Source: three-view drawing plus pictorial views. Frame: mm from the lowest corner of the part. A direction names the side the tool comes from. Round coordinates to 2 decimals unless told otherwise and drop trailing zeros. Write each loop counter-clockwise with the first axis right and the second up, starting at its lowest first coordinate (ties: lowest second). Pieces come first, ordered by that corner, then holes. Notation, with made-up numbers: (5.25, 3) - (19.25, 3) arc R9 ccw to (19.25, 7) - close; hole circle Ø11 at (19, 54). An arc over 180 degrees is marked (long way). Write each question's results on one line, items separated by ' | '.
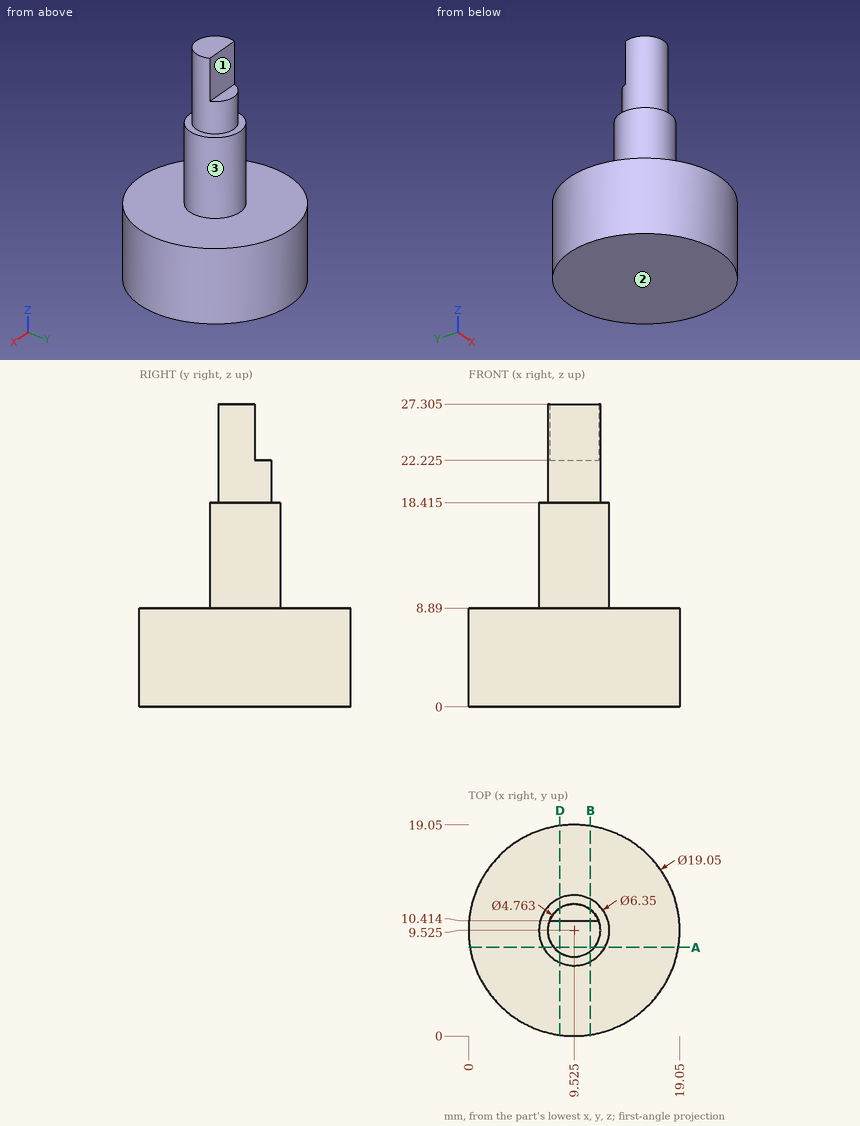
Q1. Section query D-D, the plane x = 8.25. Return loops of the section in (y, z) (1 decimal).
Answer block:
outline: (0.1, 0) - (19, 0) - (19, 8.9) - (12.4, 8.9) - (12.4, 18.4) - (11.5, 18.4) - (11.5, 22.2) - (10.4, 22.2) - (10.4, 27.3) - (7.5, 27.3) - (7.5, 18.4) - (6.6, 18.4) - (6.6, 8.9) - (0.1, 8.9) - close
Q2. Section query A-A, the plane y = 8. Return loops of the section in (x, z) (1 decimal).
Answer block:
outline: (0.1, 0) - (18.9, 0) - (18.9, 8.9) - (12.3, 8.9) - (12.3, 18.4) - (11.4, 18.4) - (11.4, 27.3) - (7.7, 27.3) - (7.7, 18.4) - (6.7, 18.4) - (6.7, 8.9) - (0.1, 8.9) - close
Q3. Access query for the marked faces 1, 2 and 3. Directions: +Z, -Z, +X, -X, +Y, -Y. A direction counts if a zero-diameter tool reaches every point of the face in a straight line with its end or side. Return the directions, or none.
Answer block:
face 1: +Z, +X, -X, +Y | face 2: -Z, +X, -X, +Y, -Y | face 3: +Z
Q4. Pin query (flat end, axial travel): pin 1 (6 mm diameter, centred on x = 4, z = 16.5, fed in from -Y); pin 2 (2 mm diameter, centred on x = 15, z = 19.5, fed in from -Y); pin 3 (3 mm diameter, centred on y = 5.5, z = 17.5, fed in from +X); pin 4 (1.2 mm diameter, centred on x = 10.5, y = 11.5, fed in from +Z) (1 decimal). Return the tip coordinate at first contact, or that it passes through.
Answer block:
pin 1: y = 7.6 | pin 2: through | pin 3: x = 11.45 | pin 4: z = 22.2
Q5. Ray query, line 1 along Z through (x, y) = (11.25, 7) (1 decimal); line 2 along Z through (x, y) = (11.5, 15.5); line 3 along X through (y, z) = (7.25, 16). Return the intervals inside material, ascending.
Answer block:
line 1: 0 to 18.4 | line 2: 0 to 8.89 | line 3: 7.31 to 11.74
Q6. Section query B-B, the plane x = 11. Return loops of the section in (y, z) (1 decimal), plus the area to 3 significant figures.
Answer block:
outline: (0.1, 0) - (18.9, 0) - (18.9, 8.9) - (12.3, 8.9) - (12.3, 18.4) - (11.4, 18.4) - (11.4, 22.2) - (10.4, 22.2) - (10.4, 27.3) - (7.7, 27.3) - (7.7, 18.4) - (6.7, 18.4) - (6.7, 8.9) - (0.1, 8.9) - close | area: 249 mm2
